Can you work these out from the drawing? Everything is in mm from the part's minimum corner. Round coordinates to 2 decimals unless told otherwise and drop trailing zeros. Loops run counter-clockwise (first coordinate to the right, second up) from the corner with the lowest first, then second, coordinate; pieces in that order, holes last. Notation, with made-up numbers: (84.5, -1) -> (103.5, -1) arc R24 cw to (103.5, 23) -> close; hole circle Ø9 at (53, 52). An arc over 180 degrees is marked (long way). One line per item, written item: value.
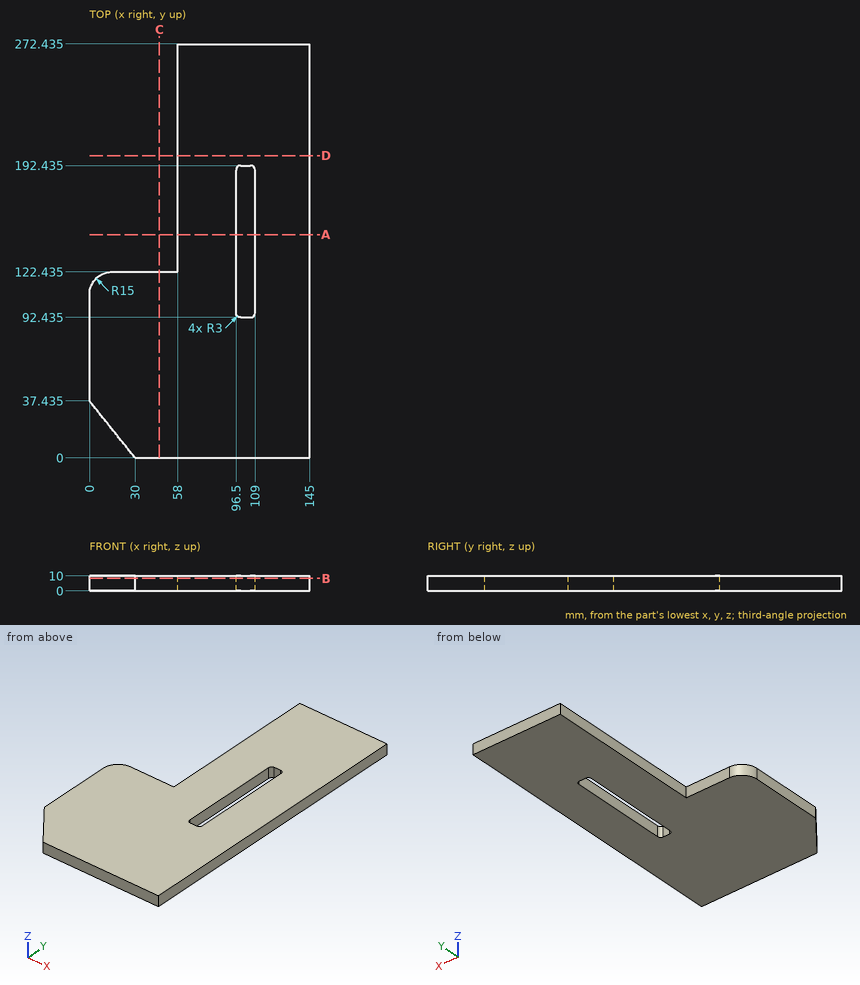
(1) If we section it at A-A, the plane y = 147: Please give me the cut outline in (x, z), then the cut area to 3 significant figures.
Recorded:
outline: (58, 0) -> (96.5, 0) -> (96.5, 10) -> (58, 10) -> close; (109, 0) -> (145, 0) -> (145, 10) -> (109, 10) -> close
area: 745 mm²
(2) I'm going to push flat-ended pins straight in: pin 1 Ø10 at (x, y) = (111.5, 84.5) entering from -Z; pin 2 Ø3 at (y, z) = (165, 2.5) entering from -X. Where does each tip first touch, or does it pass through?
Recorded:
pin 1: z = 0
pin 2: x = 58
(3) If we section it at D-D, the plane y = 199: Please give me the cut outline in (x, z).
Recorded:
outline: (58, 0) -> (145, 0) -> (145, 10) -> (58, 10) -> close
(4) If we section it at B-B, the plane z = 8.25: Please give me the cut outline in (x, y) (3 decimals).
Recorded:
outline: (0, 37.435) -> (30, 0) -> (145, 0) -> (145, 272.435) -> (58, 272.435) -> (58, 122.435) -> (15, 122.435) arc R15 ccw to (0, 107.435) -> close; hole (96.5, 95.435) arc R3 ccw to (99.5, 92.435) -> (106, 92.435) arc R3 ccw to (109, 95.435) -> (109, 189.435) arc R3 ccw to (106, 192.435) -> (99.5, 192.435) arc R3 ccw to (96.5, 189.435) -> close
(5) If I drill on L1, parallel to X at y = 144, z = 3.5; L2, parallel to Y at x = 99, z = 6.75 (3 decimals); L3, parallel to X at y = 213, z = 2.5, over which ranges is the centre line in solid material (lowest first)?
Recorded:
L1: 58 to 96.5, 109 to 145
L2: 0 to 92.477, 192.393 to 272.435
L3: 58 to 145
(6) If we section it at C-C, the plane x = 46: Please give me the cut outline in (y, z) (3 decimals).
Recorded:
outline: (0, 0) -> (122.435, 0) -> (122.435, 10) -> (0, 10) -> close
